CAD build for the part. Positions are in the model's coordinates, mm. Round coordinates to 2 decimals unless told otherwise and drop trailing zeros. Loops run counter-clockwise (first coordinate to the right, second up) from the corner with the lowest first, then second, coordinate; pieces in that order, holes last.
from build123d import *

# Parameters (mm, degrees)
SKETCH1_R               = 42.73
BOSS_EXTRUDE1_DEPTH     = 2
CUT_EXTRUDE1_DEPTH      = 61.462432965
CUT_EXTRUDE1_DEPTH_BACK = 61.462432965
SKETCH2_R               = 0.25
CUT_EXTRUDE2_DEPTH      = 61.462432965
CUT_EXTRUDE2_DEPTH_BACK = 61.462432965
SKETCH3_R               = 1


with BuildPart() as part:
    # Sketch1 → Boss-Extrude1 (new body)
    with BuildSketch(Plane(origin=(0, 0, 0), x_dir=(1, 0, 0), z_dir=(0, 1, 0))):
        with Locations(Location((0, 0, 0), (0, 0, 270))):
            Circle(SKETCH1_R)
    extrude(amount=BOSS_EXTRUDE1_DEPTH)

    # Sketch2 → Cut-Extrude1 (cut, two sides: drawn at the far end of the back side and taken through both)
    with BuildSketch(Plane(origin=(0, 2, 0), x_dir=(1, 0, 0), z_dir=(0, 1, 0)).offset(-CUT_EXTRUDE1_DEPTH_BACK)):
        with Locations(Location((0, 10.25, 0), (0, 0, 270))):
            Circle(SKETCH2_R)
    extrude(amount=CUT_EXTRUDE1_DEPTH + CUT_EXTRUDE1_DEPTH_BACK, mode=Mode.SUBTRACT)

    # Sketch3 → Cut-Extrude2 (cut, two sides: drawn at the far end of the back side and taken through both)
    with BuildSketch(Plane(origin=(0, 2, 0), x_dir=(1, 0, 0), z_dir=(0, 1, 0)).offset(-CUT_EXTRUDE2_DEPTH_BACK)):
        with Locations(Location((-11, 0, 0), (0, 0, 270))):
            Circle(SKETCH3_R)
        with Locations(Location((-7.778174593, -7.778174593, 0), (0, 0, 270))):
            Circle(SKETCH3_R)
    extrude(amount=CUT_EXTRUDE2_DEPTH + CUT_EXTRUDE2_DEPTH_BACK, mode=Mode.SUBTRACT)


solid = part.part
Item 1: Mould opens along X. For faces 1 (the cylindrical face through (-10, 1, 0)), 2 (the cylindrical face through (12.83, 0.99, 40.76)), 3 (the flat face through (1, 2, -1)) say: released by +X, released by -X, zero draft, split by the parting line, or undercut.
Verdict:
face 1: undercut
face 2: split by the parting line
face 3: zero draft
Item 2: Cut at B-B (x = -11). List the corners of the cut face in (y, z).
Verdict:
outline: (0, -41.29) - (2, -41.29) - (2, -1) - (0, -1) - close; (0, 1) - (2, 1) - (2, 41.29) - (0, 41.29) - close
Item 3: Cut at D-D (z = -21). List the corners of the cut face in (x, y), plus the area to 3 significant figures.
Verdict:
outline: (-37.21, 0) - (37.21, 0) - (37.21, 2) - (-37.21, 2) - close
area: 149 mm2
Item 4: Wall check: L1, parallel to X at y = 0.25, z = 0; L2, parallel to X at y = 0.65, z = -10.25; L3, parallel to Z at x = -11, y = 1.25. Give the ranges that are in metal, low to high.
Verdict:
L1: x = -42.73 to -12, -10 to 42.73
L2: x = -41.48 to -0.25, 0.25 to 41.48
L3: z = -41.29 to -1, 1 to 41.29
Item 5: Cut at A-A (z = 0). List the corners of the cut face in (x, y), plus the area to 3 significant figures.
Verdict:
outline: (-42.73, 0) - (-12, 0) - (-12, 2) - (-42.73, 2) - close; (-10, 0) - (42.73, 0) - (42.73, 2) - (-10, 2) - close
area: 167 mm2
Item 6: Cut at C-C (y = 0.8). List the corners of the cut face in (x, z), plus the area to 3 significant figures.
Verdict:
outline: circle Ø85.46 at (0, 0); hole circle Ø2 at (-11, 0); hole circle Ø2 at (-7.78, 7.78); hole circle Ø0.5 at (0, -10.25)
area: 5,730 mm2
